Autodesk Inventor part; units mm, degrees
ref_plane "Start Plane" through (0, 0, 0) normal (0, 0, 1) x (1, 0, 0)
ref_plane "End Plane" through (0, 0, 10) normal (0, 0, 1) x (1, 0, 0)
ref_plane "YZ Plane" through (0, 0, 0) normal (1, 0, 0) x (0, 1, 0)
ref_plane "Start Plane" through (0, 0, 0) normal (0, 0, 1) x (1, 0, 0)
ref_plane "End Plane" through (0, 0, 10) normal (0, 0, 1) x (1, 0, 0)
sketch "Sketch3" plane through (0, 0, 0) normal (0, 0, 1) x (1, 0, 0)
  line L0 (0, 0) -> (0, 10) construction
  line L1 (-10, 10) -> (-10, 0) construction
  line L2 (0, 0) -> (-10, 0) construction
  circle A0 centre (-10, 0) radius 2.1
  line L3 (-13.9007, 3.9007) -> (-6.0993, 3.9007) construction
  line L4 (-6.0993, 3.9007) -> (-6.0993, -3.9007) construction
  line L5 (-6.0993, -3.9007) -> (-13.9007, -3.9007) construction
  line L6 (-13.9007, -3.9007) -> (-13.9007, 3.9007) construction
  line L7 (-13.9007, 3.9007) -> (-6.0993, -3.9007) construction
  line L8 (-6.0993, 3.9007) -> (-13.9007, -3.9007) construction
  line L9 (-13.9007, -2.84) -> (-12.84, -3.9007) construction
  line L10 (-13.9007, -2.84) -> (-12.4007, -2.84) construction
  line L11 (-12.84, -3.9007) -> (-15.4993, -6.56)
  line L12 (-15.4993, -6.56) -> (-15.4993, -8.2)
  line L13 (-15.4993, -8.2) -> (-12.84, -8.2)
  line L14 (-12.84, -8.2) -> (-14.64, -10)
  line L15 (-7.16, -3.9007) -> (-4.5007, -6.56)
  line L16 (-4.5007, -6.56) -> (-4.5007, -8.2)
  line L17 (-4.5007, -8.2) -> (-7.16, -8.2)
  line L18 (-7.16, -8.2) -> (-5.36, -10)
  line L19 (-12.84, -3.9007) -> (-7.16, -3.9007)
  line L20 (-12.84, 3.9007) -> (-13.9007, 2.84) construction
  line L21 (-12.84, 3.9007) -> (-12.84, 2.4007) construction
  line L22 (-13.9007, 2.84) -> (-16.56, 5.4993)
  line L23 (-16.56, 5.4993) -> (-18.2, 5.4993)
  line L24 (-18.2, 5.4993) -> (-18.2, 2.84)
  line L25 (-18.2, 2.84) -> (-20, 4.64)
  line L26 (-18.2, -2.84) -> (-20, -4.64)
  line L27 (-18.2, -5.4993) -> (-18.2, -2.84)
  line L28 (-16.56, -5.4993) -> (-18.2, -5.4993)
  line L29 (-13.9007, -2.84) -> (-16.56, -5.4993)
  line L30 (-13.9007, 2.84) -> (-13.9007, -2.84)
  line L31 (-6.0993, 2.84) -> (-7.16, 3.9007) construction
  line L32 (-6.0993, 2.84) -> (-7.5993, 2.84) construction
  line L33 (-7.16, 3.9007) -> (-4.5007, 6.56)
  line L34 (-4.5007, 6.56) -> (-4.5007, 8.2)
  line L35 (-4.5007, 8.2) -> (-7.16, 8.2)
  line L36 (-7.16, 8.2) -> (-5.36, 10)
  line L37 (-12.84, 8.2) -> (-14.64, 10)
  line L38 (-15.4993, 8.2) -> (-12.84, 8.2)
  line L39 (-15.4993, 6.56) -> (-15.4993, 8.2)
  line L40 (-12.84, 3.9007) -> (-15.4993, 6.56)
  line L41 (-7.16, 3.9007) -> (-12.84, 3.9007)
  line L42 (-6.0993, 2.84) -> (-2.6993, 6.24)
  line L43 (-2.6993, 6.24) -> (-2.6993, 8.2)
  line L44 (-4.5007, 8.2) -> (0, 8.2) construction
  line L45 (-6.0993, -2.84) -> (-2.6993, -6.24)
  line L46 (-2.6993, -6.24) -> (-2.6993, -8.2)
  line L47 (10, 10) -> (10, 0) construction
  circle A1 centre (10, 0) radius 2.1
  line L48 (13.9007, 3.9007) -> (6.0993, -3.9007) construction
  line L49 (13.9007, -2.84) -> (12.84, -3.9007) construction
  line L50 (12.84, -3.9007) -> (15.4993, -6.56)
  line L51 (15.4993, -6.56) -> (15.4993, -8.2)
  line L52 (15.4993, -8.2) -> (12.84, -8.2)
  line L53 (12.84, -8.2) -> (14.64, -10)
  line L54 (7.16, -8.2) -> (5.36, -10)
  line L55 (4.5007, -8.2) -> (7.16, -8.2)
  line L56 (4.5007, -6.56) -> (4.5007, -8.2)
  line L57 (7.16, -3.9007) -> (4.5007, -6.56)
  line L58 (12.84, -3.9007) -> (7.16, -3.9007)
  line L59 (13.9007, 2.84) -> (13.9007, -2.84)
  line L60 (13.9007, 2.84) -> (16.56, 5.4993)
  line L61 (16.56, 5.4993) -> (18.2, 5.4993)
  line L62 (18.2, 5.4993) -> (18.2, 2.84)
  line L63 (18.2, 2.84) -> (20, 4.64)
  line L64 (18.2, -5.4993) -> (18.2, -2.84)
  line L65 (18.2, -2.84) -> (20, -4.64)
  line L66 (16.56, -5.4993) -> (18.2, -5.4993)
  line L67 (13.9007, -2.84) -> (16.56, -5.4993)
  line L68 (7.16, 3.9007) -> (12.84, 3.9007)
  line L69 (7.16, 3.9007) -> (4.5007, 6.56)
  line L70 (4.5007, 6.56) -> (4.5007, 8.2)
  line L71 (4.5007, 8.2) -> (7.16, 8.2)
  line L72 (7.16, 8.2) -> (5.36, 10)
  line L73 (15.4993, 8.2) -> (12.84, 8.2)
  line L74 (12.84, 8.2) -> (14.64, 10)
  line L75 (15.4993, 6.56) -> (15.4993, 8.2)
  line L76 (12.84, 3.9007) -> (15.4993, 6.56)
  line L77 (6.0993, 2.84) -> (2.6993, 6.24)
  line L78 (2.6993, 6.24) -> (2.6993, 8.2)
  line L79 (6.0993, -2.84) -> (2.6993, -6.24)
  line L80 (2.6993, -6.24) -> (2.6993, -8.2)
  line L81 (-14.64, -10) -> (-18.2, -10)
  line L82 (-20, -8.2) -> (-20, -4.64)
  line L83 (-20, 4.64) -> (-20, 8.2)
  line L84 (-18.2, 10) -> (-14.64, 10)
  line L85 (18.2, -10) -> (14.64, -10)
  line L86 (5.36, -10) -> (-5.36, -10)
  line L87 (-5.36, 10) -> (5.36, 10)
  line L88 (14.64, 10) -> (18.2, 10)
  line L89 (20, 8.2) -> (20, 4.64)
  line L90 (20, -4.64) -> (20, -8.2)
  line L91 (-2.6993, -8.2) -> (2.6993, -8.2)
  line L92 (-2.6993, 8.2) -> (2.6993, 8.2)
  line L93 (-6.0993, 2.84) -> (-6.0993, -2.84)
  line L94 (6.0993, 2.84) -> (6.0993, -2.84)
  arc A2 (-20, -8.2) -> (-18.2, -10) centre (-18.2, -8.2) ccw
  arc A3 (-18.2, 10) -> (-20, 8.2) centre (-18.2, 8.2) ccw
  arc A4 (18.2, -10) -> (20, -8.2) centre (18.2, -8.2) ccw
  arc A5 (20, 8.2) -> (18.2, 10) centre (18.2, 8.2) ccw
  point P0 (-13.9007, -3.9007)
  point P1 (-13.9007, 3.9007)
  point P2 (-13.9007, 3.9007)
  point P3 (-6.0993, 3.9007)
  point P4 (6.0993, 3.9007)
  point P5 (13.9007, -3.9007)
  point P6 (12.4007, -2.84)
  point P7 (13.9007, -3.9007)
  point P8 (13.9007, 3.9007)
  point P9 (12.84, 3.9007)
  point P10 (12.84, 2.4007)
  point P11 (13.9007, 3.9007)
  point P12 (6.0993, 3.9007)
  point P13 (7.5993, 2.84)
  point P14 (-20, 10)
  point P15 (20, -10)
  point P16 (20, 10)
  point P17 (-20, -10)
  dimension "d26" = 10
  dimension "d27" = 10
  dimension "d28" = 4.2
  dimension "d29" = 1.5
  dimension "d30" = 45
  dimension "d32" = 45
  dimension "d33" = 1.64
  dimension "d34" = 1.8
  dimension "d35" = 10
  dimension "d36" = 5.68
  dimension "d39" = 180
  dimension "d41" = 1.96
  dimension "d42" = 5.68
  dimension "d45" = 1.8
extrude "Body" add sketch "Sketch3" along normal up to surface (10 mm away) from surface at 0
sketch "Sketch4" plane through (0, 0, 0) normal (0, 0, 1) x (1, 0, 0)
  line L0 (0, 0) -> (10, 0)
ref_plane "Work Plane3" through (0, 0, 0) normal (0, -1, 0) x (1, 0, 0)
sketch "Sketch5" plane through (0, 0, 0) normal (0, -1, 0) x (1, 0, 0)
  line L0 (-28, 0) -> (28, 0)
  line L1 (-28, 10) -> (28, 10)
  dimension "d51" = 10
equation "\"d42\" = d36"
equation "\"G_OFFSET_START\" = 0"
equation "\"G_OFFSET_END\" = 0"
equation "\"G_L\" = d51"
properties part number "vslot 20 x 40" material "Aluminum 6061"
Verification items for the finished model (mm, model axes). A direction names the side the tool comes from. Give positions to 0.01 mm unless a question says otherwise; leave off trailing zeros. Loops run counter-clockwise (first coordinate to the right, second up) from the corner with the lowest first, then second, coordinate; pieces in that order, holes last. Notation, with made-up numbers: M 54.25,1.5 L 82.25,1.5 A18 ccw 82.25,18.5 Z; hole C -10,-9.5 d4. An arc over 180 degrees is marked long. Return JSON: item names as keys, results as strings.
1) Section check C-C, the plane z = 2.5. Count the separate pieces of the cut face and the enclosed holes in it, and give its area (3 significant figures).
Findings:
{"separate pieces": "1", "enclosed holes": "3", "area": "297 mm2"}
2) Mould release check, pull along X, two halves, no side actions. Record for faces 1 (the flat face through (-20, -6, 5)), 2 (the flat face through (19.09, 3.73, 4.93)), 3 (the flat face through (-6.27, 9.09, 4.93)): released by +X, released by -X, zero draft, split by the parting line, or undercut.
Findings:
{"face 1": "released by -X", "face 2": "released by +X", "face 3": "undercut"}
3) Section check A-A, the plane y = 0. Enter the section's corners in (x, z), and give its area (3 significant figures).
Findings:
{"outline": "M -13.9,0 L -12.1,0 L -12.1,10 L -13.9,10 Z; M -7.9,0 L -6.1,0 L -6.1,10 L -7.9,10 Z; M 6.1,0 L 7.9,0 L 7.9,10 L 6.1,10 Z; M 12.1,0 L 13.9,0 L 13.9,10 L 12.1,10 Z", "area": "72.0 mm2"}
4) Section check B-B, the plane x = 10. Enter the section's corners in (y, z), and give its area (3 significant figures).
Findings:
{"outline": "M -3.9,0 L -2.1,0 L -2.1,10 L -3.9,10 Z; M 2.1,0 L 3.9,0 L 3.9,10 L 2.1,10 Z", "area": "36.0 mm2"}
5) Gauge pin test, flat ends, axial feed: P1, Ø2, axis at x = -1, y = 7, coming from the +Z side; P2, Ø1.3, axis at x = -13.5, z = 6, coming from the -Y side; P3, Ø1.5, axis at y = 2, z = 3, coming from the +X side; P4, Ø3, axis at x = -9, z = 4, coming from the +Y side. Record the tip position at first contact, or that the pin passes through.
Findings:
{"P1": "passes through", "P2": "stops at y = -9.51", "P3": "stops at x = 13.9", "P4": "stops at y = 3.9"}
6) Tool access check on faces 4 (the flat face through (-15.499, 7, 5)), 5 (the flat face through (-19.09, -3.73, 4.93)), 6 (the flat face through (13.73, -9.09, 4.93)). Record the directions out of +Z, -Z, +X, -X, +Y, -Y that give a thin tool (end or side, any length) a straight path to the whole face; none if there is none.
Findings:
{"face 4": "+Z, -Z", "face 5": "+Z, -Z, -X", "face 6": "+Z, -Z, -Y"}
7) Material ranges on L1, parallel to X at y = -6.75, z = 5.25; L2, parallel to Y at x = -2.5, z = 1.25; L3, parallel to Y at x = -18, z = 2, recorded low to high. Write a range as [from, to].
Findings:
{"L1": "x = [-20, -15.5], [-4.5, -2.7], [2.7, 4.5], [15.5, 20]", "L2": "y = [-10, -8.2], [8.2, 10]", "L3": "y = [-10, -5.5], [5.5, 10]"}
8) Section check D-D, the plane x = -10.5. Enter the section's corners in (y, z).
Findings:
{"outline": "M -3.9,0 L -2.04,0 L -2.04,10 L -3.9,10 Z; M 2.04,0 L 3.9,0 L 3.9,10 L 2.04,10 Z"}
